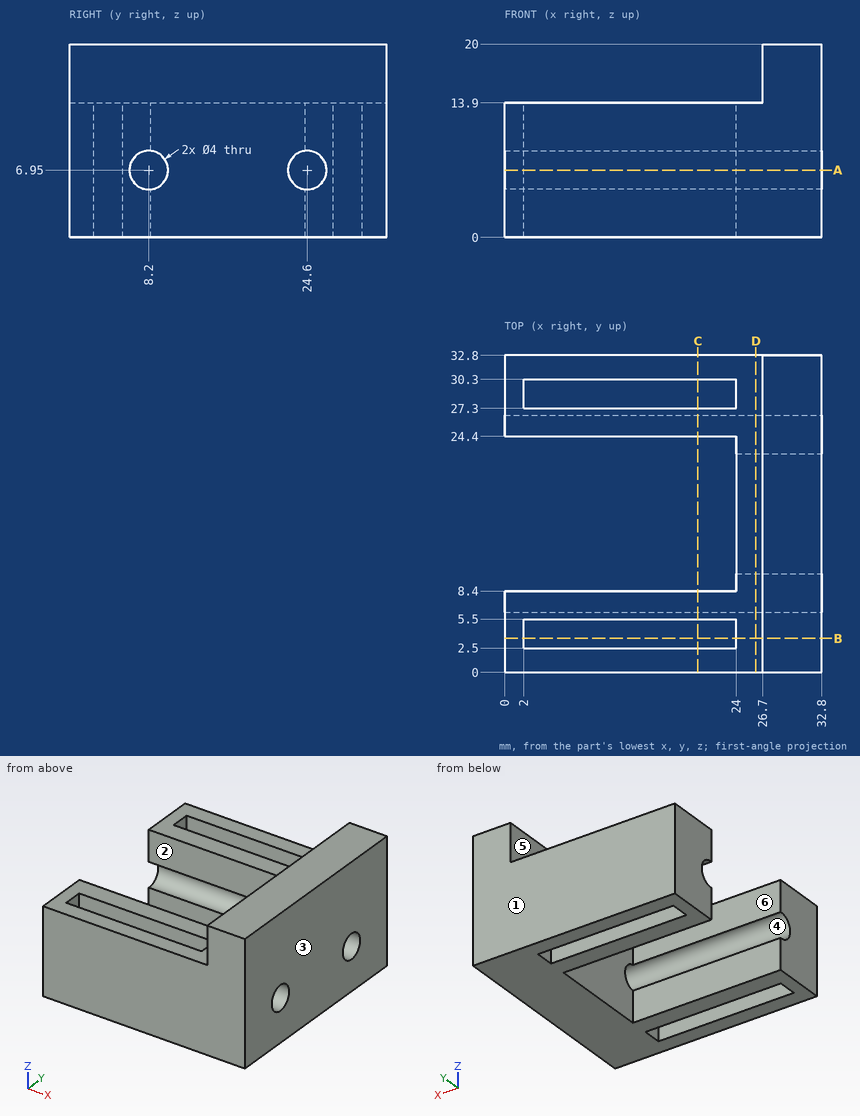
Here's the drawing with two shaded views (mm, measured from the low corner). I have some questions. A direction names the side the tool comes from. Coordinates: 2 decimals unless noted, no trailing zeros. Order: outer loops, then holes, each group sorted by start corner. A loop starts at its lowest first (then second) coordinate and runs counter-clockwise, first axis right, second up.
Item 1: If we section it at B-B, the plane y = 3.5: List the corners of the cut face in (x, z) for me, then the cut area to 3 significant figures.
Response values:
outline: (0, 0) - (2, 0) - (2, 13.9) - (0, 13.9) - close; (24, 0) - (32.8, 0) - (32.8, 20) - (26.7, 20) - (26.7, 13.9) - (24, 13.9) - close
area: 187 mm2
Item 2: Which directions (+Z, -Z, +X, -X, +Y, -Y) give clear straight access to the entire face, cutting with the end or side of a thin tool? Please do the marked faces 4, 5 and 6.
Response values:
face 4: +X, -X
face 5: +Z, -X, +Y, -Y
face 6: +Z, -Z, -X
Item 3: If we section it at A-A, the plane z = 6.95: List the corners of the cut face in (x, y) for me, then the cut area to 3 significant figures.
Response values:
outline: (0, 0) - (32.8, 0) - (32.8, 6.2) - (0, 6.2) - close; (0, 26.6) - (32.8, 26.6) - (32.8, 32.8) - (0, 32.8) - close; (24, 10.2) - (32.8, 10.2) - (32.8, 22.6) - (24, 22.6) - close; hole (2, 2.5) - (24, 2.5) - (24, 5.5) - (2, 5.5) - close; hole (2, 27.3) - (24, 27.3) - (24, 30.3) - (2, 30.3) - close
area: 384 mm2
Item 4: If we section it at C-C, the plane x = 20: List the corners of the cut face in (y, z) for me, then the cut area to 3 significant figures.
Response values:
outline: (0, 0) - (2.5, 0) - (2.5, 13.9) - (0, 13.9) - close; (5.5, 0) - (8.4, 0) - (8.4, 4.96) arc R2 cw (long way) to (8.4, 8.94) - (8.4, 13.9) - (5.5, 13.9) - close; (24.4, 0) - (27.3, 0) - (27.3, 13.9) - (24.4, 13.9) - (24.4, 8.94) arc R2 cw (long way) to (24.4, 4.96) - close; (30.3, 0) - (32.8, 0) - (32.8, 13.9) - (30.3, 13.9) - close
area: 136 mm2
Item 5: If we section it at D-D, the plane x = 26: List the corners of the cut face in (y, z) for me, then the cut area to 3 significant figures.
Response values:
outline: (0, 0) - (32.8, 0) - (32.8, 13.9) - (0, 13.9) - close; hole circle Ø4 at (8.2, 6.95); hole circle Ø4 at (24.6, 6.95)
area: 431 mm2
Item 6: I need wall thicknesses on probe 1 along Y at (x, z) = (20, 6.95); probe 2 along Y at (x, z) = (4, 2.25); probe 3 along Y at (x, z) = (29.5, 6.75). Which ranges of each line are inside material? Lowest first, please.
Response values:
probe 1: y = 0 to 2.5, 5.5 to 6.2, 26.6 to 27.3, 30.3 to 32.8
probe 2: y = 0 to 2.5, 5.5 to 8.4, 24.4 to 27.3, 30.3 to 32.8
probe 3: y = 0 to 6.21, 10.19 to 22.61, 26.59 to 32.8
Item 7: Thinking about a two-plate mould opening in Y: for the marked faces 1, 2 and 3, which applies, pulls with the +Y half, pulls with the -Y half, needs draft (parallel to the pull), parting line crosses it, or undercut?
Response values:
face 1: pulls with the +Y half
face 2: undercut
face 3: needs draft
Item 8: I'm going to push flat-ended pins straight in: pin 1 Ø6 at (y, z) = (16.5, 5.5) entering from -X; pin 2 Ø1.8 at (y, z) = (14.5, 16.5) entering from -X. Where does each tip first touch, or does it pass through?
Response values:
pin 1: stops at x = 24
pin 2: stops at x = 26.7
